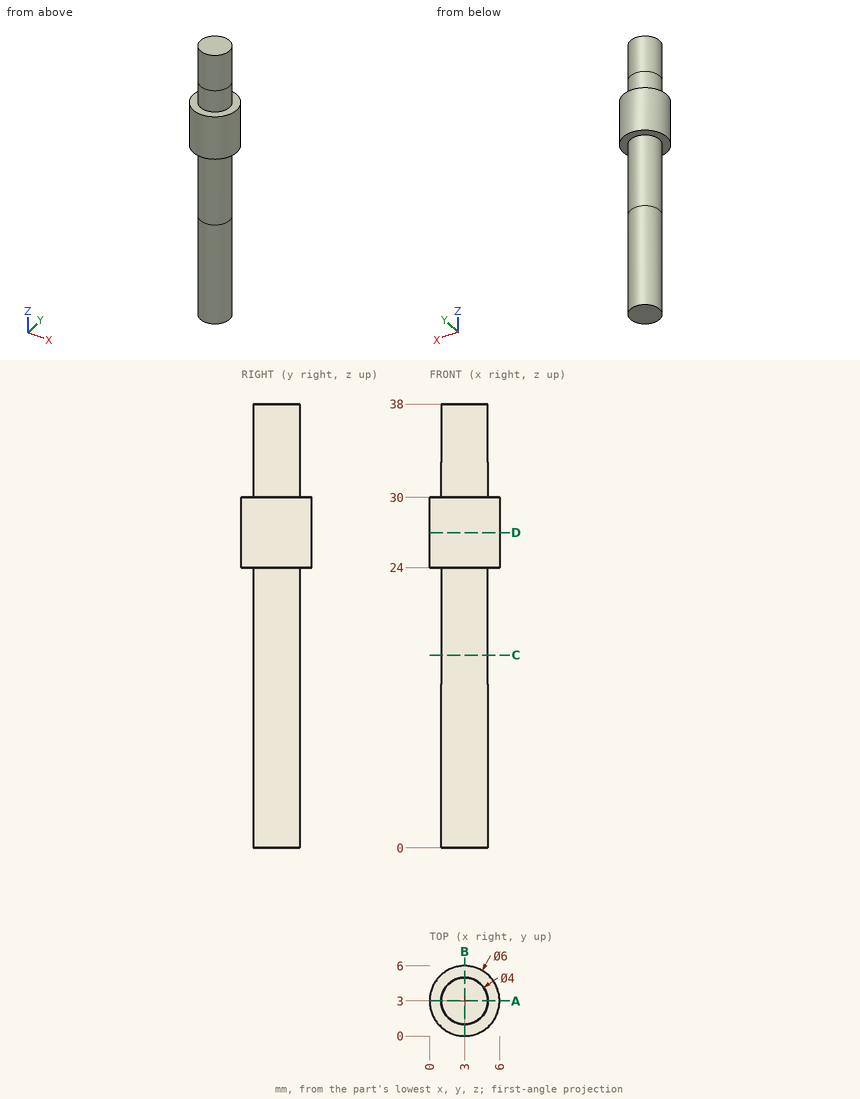
Input: dimensioned drawing with shaded views. Units: mm. Origin: part minimum x, y, z. Coordinates: 2 decimals unless noted, no trailing zeros. Loops run counter-clockwise (first coordinate to the right, second up) from the corner with the lowest first, then second, coordinate; pieces in that order, holes last. Notation, with made-up numbers: (-0.5, 34.5) -> (56.5, 34.5) arc R18 cw to (56.5, 39.5) -> close; hole circle Ø1 at (79, 75). An arc over 180 degrees is marked (long way). Use a Markdown table: item, result. Add a question column.
(1) Pin query (flat end, axial travel): pin 1 Ø2 at (x, z) = (3.5, 13.5) entering from +Y; pin 2 Ø1 at (y, z) = (4, 32) entering from -X. Return the tip coordinate at first contact, or that it passes through.
(2) Section query D-D, the plane z = 27. Return loops of the section in (x, y).
(3) Line query: line 1 along Z through (x, y) = (5.4, 3.3); line 2 along Y through (x, z) = (1.4, 21); line 3 along X through (y, z) = (4.7, 15.5). Output: solid intervals per line, ascending.
(4) Section query A-A, the plane y = 3. Return loops of the section in (x, z), plus the area to 3 significant figures.
(5) Section query C-C, the plane z = 16.5. Return loops of the section in (x, y).
Answer:
| question | item | result |
|---|---|---|
| 1 | pin 1 | stops at y = 5 |
| 1 | pin 2 | stops at x = 1.06 |
| 2 | outline | circle Ø6 at (3, 3) |
| 3 | line 1 | z = 24 to 30 |
| 3 | line 2 | y = 1.8 to 4.2 |
| 3 | line 3 | x = 1.95 to 4.05 |
| 4 | outline | (0, 24) -> (1, 24) -> (1, 0) -> (5, 0) -> (5, 24) -> (6, 24) -> (6, 30) -> (5, 30) -> (5, 38) -> (1, 38) -> (1, 30) -> (0, 30) -> close |
| 4 | area | 164 mm^2 |
| 5 | outline | circle Ø4 at (3, 3) |
